Geometry check sheet. Reference: the model listing, model coordinates, mm. A direction names the side the tool comes from. Round coordinates to 2 decimals unless told otherwise and drop trailing zeros. Loops run counter-clockwise (first coordinate to the right, second up) from the corner with the lowest first, then second, coordinate; pieces in that order, holes last. Notation, with made-up numbers: (63.25, 74.25) -> (87.25, 74.25) arc R17 ccw to (87.25, 87.25) -> close; hole circle Ø7 at (57.25, 21.25). An arc over 180 degrees is marked (long way). Use a Markdown table: item, result. Add a question column.
Q1. Gauge pin test, flat ends, axial feed: P1, Ø3, axis at x = 426, y = 151.5, coming from the -Z side; P2, Ø21, axis at x = 358.5, z = -71.5, coming from the -Y side. Record the tip position at first contact, or that the pin passes through.
Q2. Sectioned sample at A-A, the plane x = 333.5. Enter the section's corners in (y, z).
Q3. Set-up check for faces 1 (the face through (254, 350, -21)), 2 (the face through (250, 165, 76)), 3 (the face through (250, 205, 45)): record each of +Z, -Z, +X, -X, +Y, -Y from which the full face is reachable in a straight line by a thin tool's end or side.
Q4. Sectioned sample at C-C, the plane z = 9. Enter the section's corners in (x, y), then the cut area to 3 significant figures.
Q5. Sectioned sample at B-B, the plane y = 247.5. Enter the section's corners in (x, z), then the cut area to 3 significant figures.
Q6. Release check for a two-part mould opening along Y. For faces 4 (the face through (246, 203, 120)), 5 (the face through (247, 335, -70)), 6 (the face through (235, 180, 76)), 7 (the face through (250, 195, 83)) record: released by +Y, released by -Y, zero draft, split by the parting line, or undercut.
Q7. Material ranges on L1, parallel to Y at x = 243, z = 51.5; L2, parallel to Z at x = 123.5, y = 204; L3, parallel to Y at x = 394.5, z = 1, recorded low to high.
Autodesk Inventor part; units mm, degrees
ref_plane "YZ Plane" through (0, 0, 0) normal (1, 0, 0) x (0, 1, 0)
ref_plane "XZ Plane" through (0, 0, 0) normal (0, 1, 0) x (-1, 0, 0)
ref_plane "XY Plane" through (0, 0, 0) normal (0, 0, 1) x (1, 0, 0)
sketch "Sketch1" plane through (0, 0, 0) normal (1, 0, 0) x (0, 1, 0)
  line L0 (400, 120) -> (0, 120)
  line L1 (0, 40) -> (0, 62.8571)
  line L2 (400, 120) -> (0, 120)
  line L3 (0, 120) -> (0, 30)
  line L4 (0, 30) -> (400, 30)
  line L5 (400, 30) -> (400, 120)
  dimension "d54" = 400
  dimension "d55" = 90
extrude "Extrusion1" add sketch "Sketch1" along normal blind 500
sketch "Sketch2" plane through (500, 0, 0) normal (1, 0, 0) x (0, 0, -1)
  line L0 (-30, 400) -> (80, 400)
  line L1 (80, 400) -> (80, 350)
  line L2 (80, 350) -> (-30, 350)
  line L3 (-30, 350) -> (-30, 400)
  arc A0 (-42.5, 0) -> (-30, 12.5) centre (-42.5, 12.5) ccw
  line L4 (-120, 0) -> (-30, 0)
  line L5 (-30, 0) -> (-64.3382, 0)
  line L6 (-30, 12.5) -> (-30, 0)
  line L7 (-120, 400) -> (-120, 0)
  line L8 (-120, 0) -> (-70, 0)
  line L9 (-70, 0) -> (-70, 50)
  line L10 (-70, 50) -> (-120, 50)
  line L11 (-120, 50) -> (-120, 0)
  point P0 (-70, 0)
  dimension "d11" = 110
  dimension "d12" = 50
  dimension "d33" = 12.5
  dimension "d38" = 50
  dimension "d39" = 50
extrude "Extrusion11" cut sketch "Sketch2" against normal blind 500 contours A0 L6 L4
extrude "Extrusion12" add sketch "Sketch2" against normal blind 500 contours L0 L1 L2 L3
sketch "Sketch8" plane through (0, 0, 120) normal (0, 0, 1) x (1, 0, 0)
  line L0 (0, 0) -> (500, 0)
  line L1 (0, 400) -> (500, 400)
  line L2 (0, 0) -> (500, 0)
  line L3 (500, 0) -> (500, 400)
  line L4 (500, 400) -> (0, 400)
  line L5 (0, 400) -> (0, 0)
  line L6 (264, 195) -> (236, 195)
  line L7 (235, 194) -> (235, 166)
  line L8 (236, 165) -> (264, 165)
  line L9 (265, 166) -> (265, 194)
  arc A0 (236, 195) -> (235, 194) centre (236, 194) ccw
  arc A1 (265, 194) -> (264, 195) centre (264, 194) ccw
  arc A2 (264, 165) -> (265, 166) centre (264, 166) ccw
  arc A3 (235, 166) -> (236, 165) centre (236, 166) ccw
  point P0 (265, 195)
  point P1 (235, 165)
  point P2 (235, 195)
  point P3 (265, 165)
  dimension "d77" = 30
  dimension "d78" = 30
  dimension "d83" = 1
extrude "Extrusion17" cut sketch "Sketch8" against normal blind 90 contours A1 L9 A2 L8 A3 L7 A0 L6
sketch "Sketch10" plane through (500, 12.5, 30) normal (0, 0, -1) x (-1, 0, 0)
  line L0 (236, 152.5) -> (264, 152.5)
  line L1 (265, 153.5) -> (265, 201.5)
  line L2 (264, 202.5) -> (236, 202.5)
  line L3 (235, 201.5) -> (235, 153.5)
  arc A0 (236, 202.5) -> (235, 201.5) centre (236, 201.5) ccw
  arc A1 (265, 201.5) -> (264, 202.5) centre (264, 201.5) ccw
  arc A2 (264, 152.5) -> (265, 153.5) centre (264, 153.5) ccw
  arc A3 (235, 153.5) -> (236, 152.5) centre (236, 153.5) ccw
  point P0 (500, -12.5)
  point P1 (265, 202.5)
  point P2 (265, 152.5)
  point P3 (235, 202.5)
  dimension "d84" = 30
  dimension "d85" = 50
  dimension "d86" = 1
extrude "Extrusion18" cut sketch "Sketch10" against normal blind 15
fillet "Face Fillet1" radius 12.5 1 edges at (250, 350, 30)
sketch "Sketch11" plane through (0, 350, -80) normal (0, -1, 0) x (1, 0, 0)
  line L0 (500, 0) -> (0, 0)
  line L1 (500, 0) -> (0, 0)
  line L2 (0, 0) -> (0, 20)
  line L3 (0, 20) -> (500, 20)
  line L4 (500, 20) -> (500, 0)
  dimension "d92" = 500
  dimension "d93" = 20
extrude "Extrusion19" add sketch "Sketch11" along normal blind 15
fillet "Face Fillet2" radius 1 1 edges at (250, 350, -60)
fillet "Face Fillet3" radius 1 1 edges at (250, 335, -60)
properties part number "Molde" material "Aluminum 6061-AHC"
Values:
| question | item | result |
|---|---|---|
| 1 | P1 | z = 30 |
| 1 | P2 | y = 335 |
| 2 | outline | (0, 42.5) arc R12.5 ccw to (12.5, 30) -> (337.5, 30) arc R12.5 cw to (350, 17.5) -> (350, -59) arc R1 cw to (349, -60) -> (336, -60) arc R1 ccw to (335, -61) -> (335, -80) -> (400, -80) -> (400, 120) -> (0, 120) -> close |
| 3 | face 1 | +X, -X, -Y |
| 3 | face 2 | +Z, -Z |
| 3 | face 3 | -Z |
| 4 | outline | (0, 350) -> (500, 350) -> (500, 400) -> (0, 400) -> close |
| 4 | area | 25,000 mm^2 |
| 5 | outline | (0, 30) -> (500, 30) -> (500, 120) -> (0, 120) -> close |
| 5 | area | 45,000 mm^2 |
| 6 | face 4 | zero draft |
| 6 | face 5 | released by -Y |
| 6 | face 6 | undercut |
| 6 | face 7 | undercut |
| 7 | L1 | 0 to 165, 195 to 400 |
| 7 | L2 | 30 to 120 |
| 7 | L3 | 350 to 400 |
